Answer from the drawing. Dimensions are ordinates in mm from the lowest x, y and z of the part. A direction names the side the tool comes from. Give positions to 0.01 mm unless a question says otherwise; leave off trailing zeros. Order: outer loops, then holes, each group sorted by start corner. A loop starts at its lowest first (then second) coordinate and runs counter-clockwise, first axis right, second up. Notation, with made-up numbers: (42.25, 83.5) -> (72.25, 83.5) arc R23 cw to (72.25, 122.5) -> close; hole circle Ø11 at (-16.5, -32). An arc over 180 degrees is marked (long way). Answer as a JSON object with one key per item and string values. Group by question number.
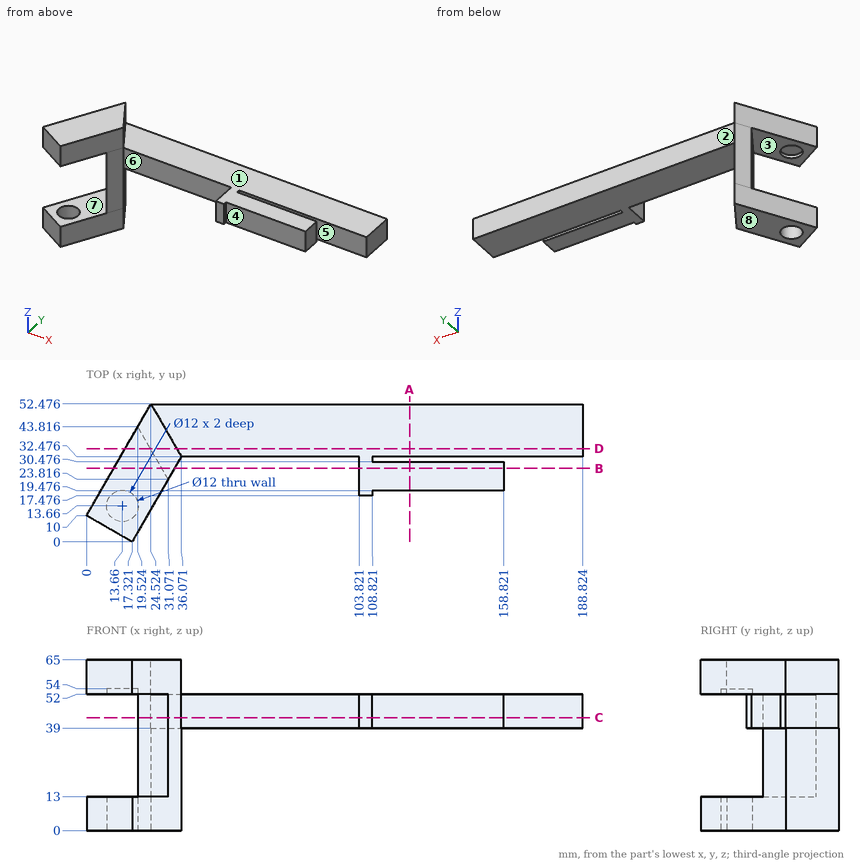
(1) For a pull along Z with two mould halves and no side action, classify the marked faces 1, 2 and 3 as +Z half, -Z half, draft (parallel to the pull), parting line (faces both ways), or undercut.
(2) Find the intervals of material crossed by line 1 along X through (y, z) = (20, 46.5); line 2 along Z through (x, y) = (171, 37); line 3 along X through (y, z) = (36, 8) (1 decimal), in increasing order. Write a range as [from, to].
(3) Flat-ended cylindrical pins translate along their axes: pin 1 Ø2 at (y, z) = (46, 56.5) entering from +X; pin 2 Ø5.5 at (x, z) = (106.5, 48) entering from -Y; pin 3 Ø4 at (x, z) = (132, 48.5) entering from -Y. Find the tip coordinate at first contact, or state that the pin passes through.
(4) A cutting plane is placed at C-C (z = 43). Determine the outline of the cut face in (x, y) (1 decimal).
(5) A cutting plane is placed at A-A (x = 123). Determine the outline of the cut face in (y, z) (1 decimal), and give its area (3 significant figures).
(6) A cutting plane is placed at D-D (y = 35.5). Determine the outline of the cut face in (x, z) (1 decimal).
(7) Which of the six approach directions +Z, -Z, +X, -X, +Y, -Y give full straight-line access (tool end or side, diameter ignored) to the marked faces 4, 5, 6, 7 and 8?
(8) A cutting plane is placed at B-B (y = 28). Determine the outline of the cut face in (x, z) (1 decimal).
Check sheet entries:
{
 "1": {"face 1": "+Z half", "face 2": "draft", "face 3": "undercut"},
 "2": {"line 1": "x = [103.82, 158.82]", "line 2": "z = [39, 52]", "line 3": "x = [15, 34]"},
 "3": {"pin 1": "stops at x = 28.84", "pin 2": "stops at y = 17.48", "pin 3": "stops at y = 19.48"},
 "4": {"outline": "(19.5, 43.8) -> (31.1, 23.8) -> (36.1, 32.5) -> (103.8, 32.5) -> (103.8, 17.5) -> (108.8, 17.5) -> (108.8, 19.5) -> (158.8, 19.5) -> (158.8, 30.5) -> (108.8, 30.5) -> (108.8, 32.5) -> (188.8, 32.5) -> (188.8, 52.5) -> (24.5, 52.5) -> close"},
 "5": {"outline": "(19.5, 39) -> (30.5, 39) -> (30.5, 52) -> (19.5, 52) -> close; (32.5, 39) -> (52.5, 39) -> (52.5, 52) -> (32.5, 52) -> close", "area": "403 mm2"},
 "6": {"outline": "(14.7, 0) -> (34.3, 0) -> (34.3, 39) -> (188.8, 39) -> (188.8, 52) -> (34.3, 52) -> (34.3, 65) -> (14.7, 65) -> (14.7, 52) -> (24.3, 52) -> (24.3, 13) -> (14.7, 13) -> close"},
 "7": {"face 4": "+Z, -Z, +X, -Y", "face 5": "+Z, -Z, +X", "face 6": "+Z, -Z, -Y", "face 7": "-X, -Y", "face 8": "-Z, +X, -X, +Y, -Y"},
 "8": {"outline": "(10.4, 0) -> (33.5, 0) -> (33.5, 65) -> (10.4, 65) -> (10.4, 52) -> (28.7, 52) -> (28.7, 13) -> (10.4, 13) -> close; (103.8, 39) -> (158.8, 39) -> (158.8, 52) -> (103.8, 52) -> close"}
}
